The listing builds one solid part. Answer for the finished solid, in the listing's coordinates (mm). Coordinates: 2 decimals unless noted, no trailing zeros. Loops run counter-clockwise (first coordinate to the right, second up) from the corner with the lowest first, then second, coordinate; pieces in that order, holes last. Notation, with made-up numbers: M 7,-29.75 L 19,-29.75 A20 ccw 19,-19.75 Z; hole C 40.5,5.5 d1. An arc over 180 degrees is marked long. Return JSON: item names as keys, results as strings. Group by question number.
1. Section A-A (x = 0) is taken. Write down the section's boundary in (y, z), then the cut area to 3 significant figures.
2. Given P1, Ø3.5, axis at x = -6, z = 1, coming from the -Y side; P2, Ø1.5, axis at y = 4.5, z = -24.5, coming from the -X side; P3, Ø3, axis at y = 3.5, z = -3.5, coming from the +X side, each flat-ended and moving along its own axis, determine where each tip first touches the part or whether it passes through.
3. Straight lines are drawn through the part: L1, parallel to X at y = 2.9, z = 0; L2, parallel to Y at x = 7, z = -2.5. For each, find the intervals that lie inside material, in ascending order. Write a range as from..to.
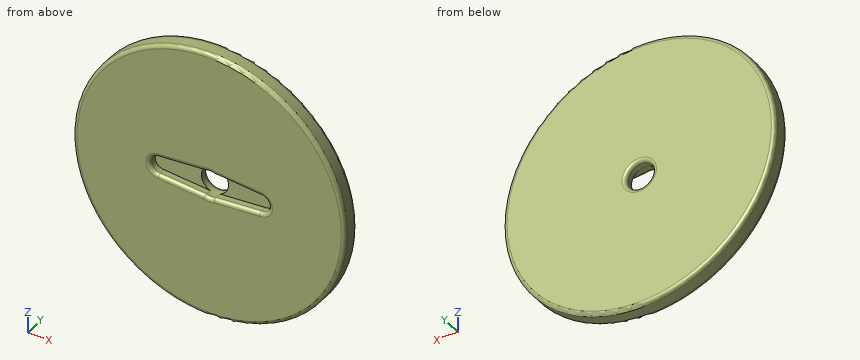
```python
from build123d import *

# Parameters (mm, degrees)
SKETCH1_R           = 37.5
SKETCH1_R_2         = 3.75
BOSS_EXTRUDE1_DEPTH = 5
CUT_EXTRUDE1_DEPTH  = 2.5
FILLET1_R           = 1


with BuildPart() as part:
    # Sketch1 → Boss-Extrude1 (new body)
    with BuildSketch(Plane(origin=(0, 0, 0), x_dir=(1, 0, 0), z_dir=(0, 1, 0))):
        Circle(SKETCH1_R)
        Circle(SKETCH1_R_2, mode=Mode.SUBTRACT)
    extrude(amount=BOSS_EXTRUDE1_DEPTH)

    # Sketch2 → Cut-Extrude1 (cut)
    with BuildSketch(Plane.XZ):
        with BuildLine():
            Line((-14, 2.5), (-1.226116774, 3.543887365))
            ThreePointArc((-1.226116774, 3.543887365), (0, 3.75), (1.226116774, 3.543887365))
            Line((1.226116774, 3.543887365), (14, 2.5))
            ThreePointArc((14, 2.5), (16.5, 0), (14, -2.5))
            Line((14, -2.5), (1.307857892, -3.514542322))
            ThreePointArc((1.307857892, -3.514542322), (0, -3.75), (-1.307857892, -3.514542322))
            Line((-1.307857892, -3.514542322), (-14, -2.5))
            ThreePointArc((-14, -2.5), (-16.5, 0), (-14, 2.5))
        make_face()
    extrude(amount=-CUT_EXTRUDE1_DEPTH, mode=Mode.SUBTRACT)

    # Fillet1
    fillet1_edges = [part.edges().sort_by_distance(p)[0] for p in [
        (0, 0, 3.75),
        (7.653928946, 0, -3.007271161),
        (16.5, 0, 0),
        (-37.5, 0, 0),
        (7.613058387, 0, 3.021943683),
        (-7.613058387, 0, 3.021943683),
        (-16.5, 0, 0),
        (-7.653928946, 0, -3.007271161),
        (-37.5, 5, 0),
        (-3.75, 5, 0),
        (0, 0, -3.75),
    ]]
    fillet(fillet1_edges, radius=FILLET1_R)


solid = part.part
```
Worked out:
{
 "1": {"outline": "M 0,-36.5 A1 ccw 1,-37.5 L 4,-37.5 A1 ccw 5,-36.5 L 5,-4.75 A1 ccw 4,-3.75 L 1,-3.75 A1 ccw 0,-4.75 Z; M 0,4.75 A1 ccw 1,3.75 L 4,3.75 A1 ccw 5,4.75 L 5,36.5 A1 ccw 4,37.5 L 1,37.5 A1 ccw 0,36.5 Z", "area": "336 mm^2"},
 "2": {"P1": "y = 2.5", "P2": "x = -28.94", "P3": "x = 37.45"},
 "3": {"L1": "-37.5..-3.75, 3.75..37.5", "L2": "2.5..5"}
}
